CAD build for the part. Positions are in the model's coordinates, mm. Face numbers are marked on the shaded views. A direction names the side the tool comes from. Round coordinates to 2 decimals unless told otherwise and drop trailing zeros. Order: outer loops, then holes, each group sorted by start corner. A loop starts at its lowest first (then second) coordinate and runs counter-clockwise, first axis right, second up. Notation, with made-up numbers: M 47,81.25 L 94,81.25 A31 cw 94,120.25 Z; hole C 86.5,-18.5 d1. An arc over 180 degrees is marked long. Answer as a JSON object with one key per item and string values.
```python
from build123d import *

# Parameters (mm, degrees)
BOSS_EXTRUDE1_DEPTH     = 44
CUT_EXTRUDE1_DEPTH      = 46
CUT_EXTRUDE1_DEPTH_BACK = 2
BOSS_EXTRUDE3_DEPTH     = 3
BOSS_EXTRUDE4_DEPTH     = 3


with BuildPart() as part:
    # Sketch2 → Boss-Extrude1 (new body)
    with BuildSketch(Plane(origin=(0, 0, 0), x_dir=(1, 0, 0), z_dir=(0, 1, 0))):
        with BuildLine():
            Line((0, 27), (46, 27))
            ThreePointArc((46, 27), (73, 0), (46, -27))
            Line((46, -27), (0, -27))
            ThreePointArc((0, -27), (-27, 0), (0, 27))
        make_face()
    extrude(amount=BOSS_EXTRUDE1_DEPTH)

    # Sketch3 → Cut-Extrude1 (cut, two sides)
    with BuildSketch(Plane(origin=(0, 0, 0), x_dir=(1, 0, 0), z_dir=(0, 1, 0))) as cut_extrude1_sk:
        with BuildLine():
            Line((0, 25.059391222), (45.856281638, 25.059391222))
            ThreePointArc((45.856281638, 25.059391222), (70.91567286, 0), (45.856281638, -25.059391222))
            Line((45.856281638, -25.059391222), (0, -25.059391222))
            ThreePointArc((0, -25.059391222), (-25.059391222, 0), (0, 25.059391222))
        make_face()
    extrude(amount=CUT_EXTRUDE1_DEPTH, mode=Mode.SUBTRACT)
    extrude(cut_extrude1_sk.sketch, amount=-CUT_EXTRUDE1_DEPTH_BACK, mode=Mode.SUBTRACT)

    # Sketch4 → Boss-Extrude3 (add)
    with BuildSketch(Plane(origin=(0, 0, 0), x_dir=(1, 0, 0), z_dir=(0, 1, 0))):
        with BuildLine():
            Line((0, 27), (46, 27))
            ThreePointArc((46, 27), (73, 0), (46, -27))
            Line((46, -27), (0, -27))
            ThreePointArc((0, -27), (-27, 0), (0, 27))
        make_face()
    extrude(amount=-BOSS_EXTRUDE3_DEPTH)

    # Sketch5 → Boss-Extrude4 (add)
    with BuildSketch(Plane(origin=(0, 0, 0), x_dir=(1, 0, 0), z_dir=(0, 1, 0))):
        Polygon((-13.939721019, 10.08564224), (-13.939721019, 4.695281904), (-15.675819956, 4.695281904), (-15.675819956, 11.794197793), (-9.286795656, 11.794197793), (-9.286795656, 10.08564224), align=None)
        Polygon((26.347826906, -10.126495255), (26.347826906, -4.736134919), (28.083925843, -4.736134919), (28.083925843, -11.835050808), (21.694901543, -11.835050808), (21.694901543, -10.126495255), align=None)
    extrude(amount=BOSS_EXTRUDE4_DEPTH)


solid = part.part
```
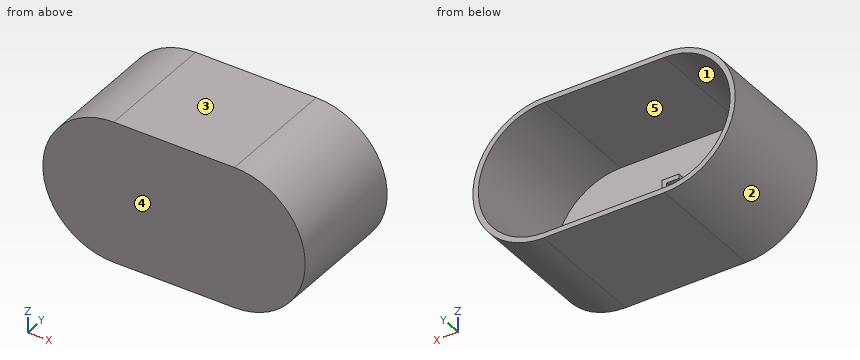
Item 1: Saw through at B-B on z = 0. List the corners of the cut face in (x, y), and give its area (3 significant figures).
Worked answers:
{"outline": "M -27,-3 L 73,-3 L 73,44 L 70.92,44 L 70.92,0 L -25.06,0 L -25.06,44 L -27,44 Z", "area": "477 mm2"}
Item 2: Saw through at C-C on x = 23. List the corners of the cut face in (y, z).
Worked answers:
{"outline": "M -3,-27 L 44,-27 L 44,-25.06 L 0,-25.06 L 0,10.13 L 3,10.13 L 3,11.84 L 0,11.84 L 0,25.06 L 44,25.06 L 44,27 L -3,27 Z"}
Item 3: 3-axis set-ups, long thin cutter, end or side, ignore diameter. For the marked faces 1 and 2: which of +Z, -Z, +X, -X, +Y, -Y reach the whole face in a straight line?
Worked answers:
{"face 1": "+Y", "face 2": "-X, +Y, -Y"}
Item 4: Two-plate mould, pull along Z, no slides. Class the marked faces 3, 4 and 5: released by +Z, released by -Z, zero draft, split by the parting line, or undercut.
Worked answers:
{"face 3": "released by +Z", "face 4": "zero draft", "face 5": "undercut"}
Item 5: Wall check: line 1 along Z through (x, y) = (33, 6.5); line 2 along Z through (x, y) = (46.5, 32.5); line 3 along Y through (x, z) = (-19.5, 5.5). Give the ranges that are in metal, low to high. Write a range as [from, to].
Worked answers:
{"line 1": "z = [-27, -25.06], [25.06, 27]", "line 2": "z = [-27, -25.05], [25.05, 27]", "line 3": "y = [-3, 0]"}
Item 6: Saw through at D-D on x = 13. List the corners of the cut face in (y, z).
Worked answers:
{"outline": "M -3,-27 L 44,-27 L 44,-25.06 L 0,-25.06 L 0,25.06 L 44,25.06 L 44,27 L -3,27 Z"}
Item 7: Saw through at A-A on y = 15.5. List the corners of the cut face in (x, z), and give its area (3 significant figures).
Worked answers:
{"outline": "M 0,-27 L 46,-27 A27 ccw 46,27 L 0,27 A27 ccw Z; hole M 0,-25.06 L 45.86,-25.06 A25.06 ccw 45.86,25.06 L 0,25.06 A25.06 ccw Z", "area": "503 mm2"}
Item 8: Drop flat-ended pins along their axis: pin 1 Ø1.4 at (y, z) = (1.5, 11) entering from -X; pin 2 Ø3.5 at (y, z) = (1, 8) entering from +X; pin 3 Ø12 at (y, z) = (4.5, 12.5) entering from +X. Give the stop position or say it passes through.
Worked answers:
{"pin 1": "stops at x = -24.96", "pin 2": "stops at x = 72.27", "pin 3": "stops at x = 72.21"}
